from build123d import *

# Parameters (mm, degrees)
SKETCH1_R           = 3.175
EXTRUDE1_DEPTH      = 102.108
SKETCH2_R           = 1
EXTRUDE2_DEPTH      = 6.35
SKETCH4_R           = 1.35382
BOSS_EXTRUDE2_DEPTH = 6.35
SKETCH5_R           = 2.3114
BOSS_EXTRUDE3_DEPTH = 2.8448


with BuildPart() as part:
    # Sketch1 → Extrude1 (new body)
    with BuildSketch(Plane(origin=(0, 0, 0), x_dir=(1, 0, 0), z_dir=(0, 1, 0))):
        with Locations(Location((0, 0, 0), (0, 0, 270))):  # turned: the seam where the file's is
            Circle(SKETCH1_R)
    extrude(amount=EXTRUDE1_DEPTH)

    # Sketch2 → Extrude2 (cut)
    with BuildSketch(Plane.XZ):
        with Locations(Location((0, 0, 0), (0, 0, 270))):  # turned: the seam where the file's is
            Circle(SKETCH2_R)
    extrude(amount=-EXTRUDE2_DEPTH, mode=Mode.SUBTRACT)

    # Sketch4 → Boss-Extrude2 (add)
    with BuildSketch(Plane.XY):
        with Locations(Location((0, 4.85382, 0), (0, 0, 180))):  # turned: the seam where the file's is
            Circle(SKETCH4_R)
    extrude(amount=BOSS_EXTRUDE2_DEPTH)

    # Sketch5 → Boss-Extrude3 (add)
    with BuildSketch(Plane.XY.offset(6.35)):
        with Locations((0, 4.85382)):
            Circle(SKETCH5_R)
    extrude(amount=BOSS_EXTRUDE3_DEPTH)


solid = part.part
Read the model definition and answer for the solid it produces. Units are mm, in the model's axes. A direction names the side the tool comes from. Round coordinates to 2 decimals unless told otherwise and drop trailing zeros. Loops run counter-clockwise (first coordinate to the right, second up) from the corner with the lowest first, then second, coordinate; pieces in that order, holes last. Notation, with made-up numbers: (-35, 76.5) - (-10, 76.5) arc R17 cw to (-10, 90.5) - close; hole circle Ø6 at (2, -19). An arc over 180 degrees is marked (long way). One line per question, with ' | ' between items. Start each with the question number.
Q1. For a pull along X with two mould halves and no side action, classify faces 4 (the flat face through (1, 0, -1)), 5 (the cylindrical face through (0.14, 50.34, -3.17)), 6 (the cylindrical face through (0, 2, -1)) as +X half, -X half, draft (parallel to the pull), parting line (faces both ways), or undercut.
Q2. For faces 1 (the cylindrical face through (-0.501, 2.597, 7.752)), 2 (the flat face through (0, 3, 6.35)), 3 (the flat face through (0, 102.108, 0)), determine the directions among +Z, -Z, +X, -X, +Y, -Y from which every point of the face is accessible in a straight line to the end or side of a thin tool.
Q3. Section B-B on y = 35 is taken. Give the vertices of the cut face in (x, z) (3 decimals), plus the area to 3 significant figures.
Q4. Flat-ended cylindrical pins translate along their axes: pin 1 (2 mm diameter, centred on x = 2, y = 12.5, fed in from -Z); pin 2 (0.6 mm diameter, centred on x = 0, z = 0, fed in from -Y); pin 3 (1.5 mm diameter, centred on y = 82.5, z = 3.5, fed in from +X). Find the tip coordinate at first contact, or state that the pin passes through.
Q5. Section A-A on x = 0 is taken. Give the vertices of the cut face in (y, z) (3 decimals), plus the area to 3 significant figures.
Q6. Find the intervals of material crossed by L1, parallel to X at y = 2.25, z = 0 (3 decimals); L2, parallel to Y at x = -1, z = 6; L3, parallel to Z at x = 0.75, y = 36, in increasing order.
Established:
1) face 4: draft | face 5: parting line | face 6: undercut
2) face 1: +Z | face 2: none | face 3: +Z, -Z, +X, -X, +Y
3) outline: circle Ø6.35 at (0, 0) | area: 31.7 mm²
4) pin 1: z = -3.01 | pin 2: y = 3.5 | pin 3: x = 1.59
5) outline: (0, -3.175) - (102.108, -3.175) - (102.108, 3.175) - (6.208, 3.175) - (6.208, 6.35) - (7.165, 6.35) - (7.165, 9.195) - (2.542, 9.195) - (2.542, 6.35) - (3.5, 6.35) - (3.5, 3.175) - (0, 3.175) - (0, 1) - (3.5, 1) - (3.5, 0) - (6.208, 0) - (6.208, 1) - (6.35, 1) - (6.35, -1) - (0, -1) - close | area: 660 mm²
6) L1: -3.175 to -1, 1 to 3.175 | L2: 3.94 to 5.77 | L3: -3.09 to 3.09
